Design review of the part shown in the three views and the two pictorial views. Dimensions are in mm from the part's minimum x, y and z. A direction names the side the tool comes from. Round coordinates to 2 decimals unless told otherwise and drop trailing zeros. Loops run counter-clockwise (first coordinate to the right, second up) from the corner with the lowest first, then second, coordinate; pieces in that order, holes last. Notation, with made-up numbers: (-22, -37.75) - (-14, -37.75) arc R27 cw to (-14, -19.75) - close; hole circle Ø1 at (88, 5). An arc over 180 degrees is marked (long way). Return JSON: item names as keys, results as strings. Group by question number.
(1) We need section C-C, the plane y = 93. Write out the cut boundary in (x, z) (1 decimal).
(2) The part is to be moulded in two halves that separate along X. For the marked faces 6, 7 and 8, say which applies: pulls with the +X half, pulls with the -X half, needs draft (parallel to the pull), parting line crosses it, or undercut.
(3) We need section B-B, the plane z = 62. Write out the cut boundary in (x, y) (1 decimal), and give its area (3 significant figures).
(4) We need section D-D, the plane y = 47. Write out the cut boundary in (x, z) (1 decimal).
(5) Clearance check with flat-ended pins moving along their axes: pin 1 (1.5 mm diameter, centred on x = 27, y = 75, fed in from +Z); pin 2 (12 mm diameter, centred on y = 84, z = 137.5, fed in from +X); pin 3 (6 mm diameter, centred on x = 129.5, y = 31.5, fed in from -Z). State where each tip first meets the part, or that it passes through.
(6) We need section A-A, the plane x = 94. Write out the cut boundary in (y, z) (1 decimal), and give its area (3 significant figures).
(7) Wall thickness on L1, parallel to Z at x = 82.5, y = 69.5; L2, parallel to X at y = 64, z = 26; L3, parallel to X at y = 74.5, z = 11: over which ranges is each line inside the solid? List them lowest first. Write a range as [from, to].
(8) For the marked faces 1, 2, 3, 4 and 5, list the 3-axis set-ups (+Z, -Z, +X, -X, +Y, -Y) from which the entire face can be reached by the end or side of a thin tool; tool diameter is ignored.
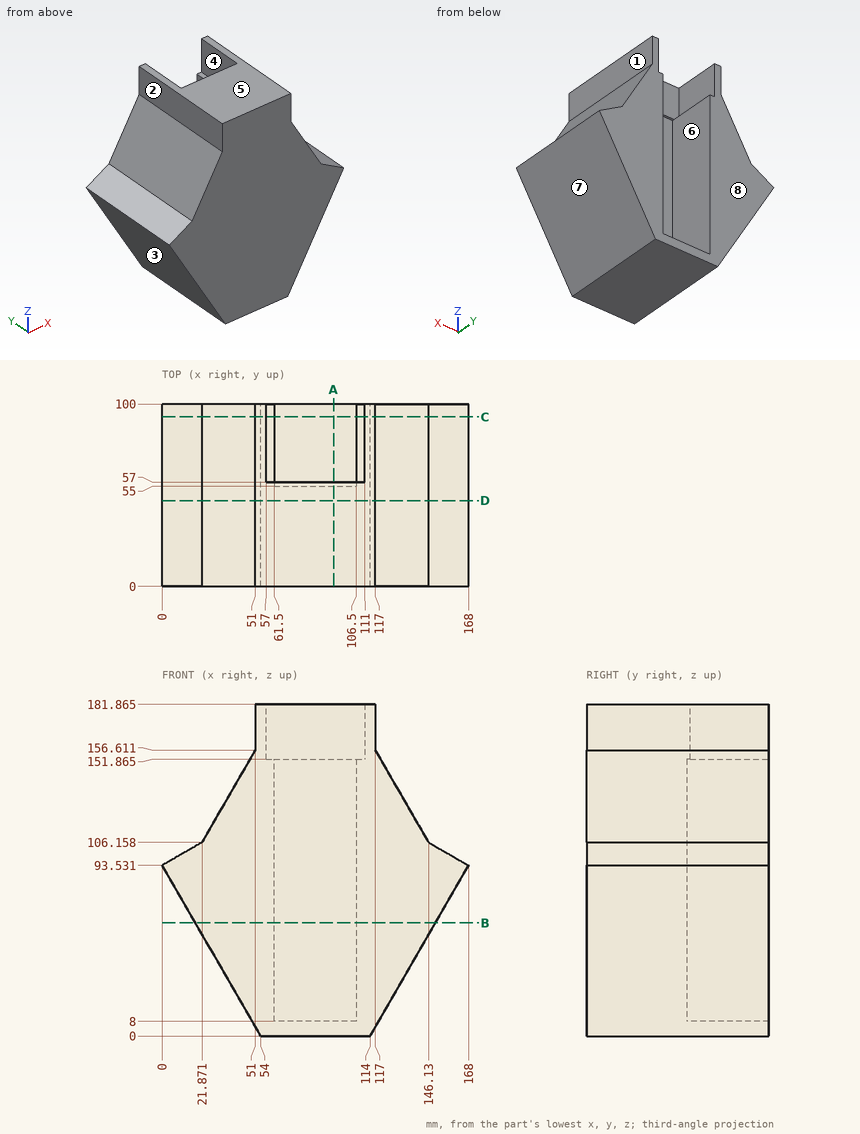
Solutions:
{
 "1": {"outline": "(0, 93.5) - (54, 0) - (114, 0) - (168, 93.5) - (146.1, 106.2) - (117, 156.6) - (117, 181.9) - (111, 181.9) - (111, 151.9) - (106.5, 151.9) - (106.5, 8) - (61.5, 8) - (61.5, 151.9) - (57, 151.9) - (57, 181.9) - (51, 181.9) - (51, 156.6) - (21.9, 106.2) - close"},
 "2": {"face 6": "undercut", "face 7": "pulls with the +X half", "face 8": "needs draft"},
 "3": {"outline": "(18.2, 0) - (149.8, 0) - (149.8, 100) - (106.5, 100) - (106.5, 55) - (61.5, 55) - (61.5, 100) - (18.2, 100) - close", "area": "11,100 mm^2"},
 "4": {"outline": "(0, 93.5) - (54, 0) - (114, 0) - (168, 93.5) - (146.1, 106.2) - (117, 156.6) - (117, 181.9) - (51, 181.9) - (51, 156.6) - (21.9, 106.2) - close"},
 "5": {"pin 1": "z = 116.34", "pin 2": "x = 131.5", "pin 3": "z = 21.65"},
 "6": {"outline": "(0, 0) - (100, 0) - (100, 8) - (55, 8) - (55, 151.9) - (57, 151.9) - (57, 181.9) - (0, 181.9) - close", "area": "10,400 mm^2"},
 "7": {"L1": "[0, 8]", "L2": "[38.99, 61.5], [106.5, 129.01]", "L3": "[47.65, 61.5], [106.5, 120.35]"},
 "8": {"face 1": "+Z, +X, +Y, -Y", "face 2": "+Z, -X, +Y, -Y", "face 3": "-Z, -X, +Y, -Y", "face 4": "+Z, +Y", "face 5": "+Z, +X, -X, +Y, -Y"}
}
